Source: CAD feature listing. Evaluate the final solid. Frame: model axes, mm. Coordinates: 2 decimals unless noted, no trailing zeros. Order: outer loops, then holes, each group sorted by start corner. A loop starts at its lowest first (then second) coordinate and runs counter-clockwise, first axis right, second up.
```python
from build123d import *

# Parameters (mm, degrees)
SKETCH1_R           = 25
BOSS_EXTRUDE1_DEPTH = 3
CUT_EXTRUDE1_DEPTH  = 0.1


with BuildPart() as part:
    # Sketch1 → Boss-Extrude1 (new body)
    with BuildSketch(Plane(origin=(0, 0, 0), x_dir=(0, 1, 0), z_dir=(0, 0, 1))):
        with Locations(Location((0, 0, 0), (0, 0, 270))):
            Circle(SKETCH1_R)
    extrude(amount=BOSS_EXTRUDE1_DEPTH)

    # Sketch3 → Cut-Extrude1 (cut)
    # profile 1 of 2: a face of its own
    with BuildSketch(Plane.XY.offset(3)):
        with BuildLine():
            Line((-2.135536589, -3.91952773), (-2.135536589, -5.589026656))
            Line((-2.135536589, -5.589026656), (-9.359581237, -5.589026656))
            Line((-9.359581237, -5.589026656), (-9.359581237, -3.91952773))
            Line((-9.359581237, -3.91952773), (-6.712942094, -3.91952773))
            Line((-6.712942094, -3.91952773), (-6.712942094, 3.6938054))
            add(Edge.make_bspline(
                [(-6.712942094, 3.6938054), (-6.711155885, 3.847105408), (-6.707541754, 4.157285237), (-6.693777105, 4.467181218), (-6.686815351, 4.623917478)],
                knots=[0, 0, 0, 0, 0.98845891, 2, 2, 2, 2], degree=3))
            Line((-6.686815351, 4.623917478), (-8.565328227, 3.051087504))
            add(Edge.make_bspline(
                [(-8.565328227, 3.051087504), (-8.617759942, 3.014331802), (-8.716372329, 2.945202508), (-8.880339811, 2.88896631), (-9.036125684, 2.875345654), (-9.18237461, 2.882130045), (-9.313965386, 2.925554364), (-9.431240682, 2.977107644), (-9.527057416, 3.04704147), (-9.573128253, 3.104942057), (-9.594721931, 3.132080409)],
                knots=[0, 0, 0, 0, 1.335478134, 2.511737127, 3.574879376, 4.598514131, 5.550291057, 6.455707661, 7.276180923, 8, 8, 8, 8], degree=3))
            Line((-9.594721931, 3.132080409), (-10.297531338, 4.098769928))
            Line((-10.297531338, 4.098769928), (-6.315815589, 7.484795919))
            Line((-6.315815589, 7.484795919), (-4.484330852, 7.484795919))
            Line((-4.484330852, 7.484795919), (-4.484330852, -3.91952773))
            Line((-4.484330852, -3.91952773), (-2.135536589, -3.91952773))
        make_face()
    # profile 2 of 2: a face of its own
    with BuildSketch(Plane.XY.offset(3)):
        with BuildLine():
            add(Edge.make_bspline(
                [(9.075449156, 0.940046608), (9.071019121, 0.664701426), (9.062453061, 0.132285105), (8.994417033, -0.639500558), (8.881176325, -1.355733726), (8.722500681, -2.017311728), (8.521457839, -2.6215582), (8.285804124, -3.171554325), (8.017952132, -3.668932341), (7.711163277, -4.110013082), (7.372230822, -4.49674732), (7.00440566, -4.832496752), (6.604657821, -5.113627074), (6.176960126, -5.341859495), (5.726135225, -5.515862981), (5.257991212, -5.64302657), (4.771230439, -5.71676622), (4.440808731, -5.727356618), (4.273353654, -5.732723747)],
                knots=[0, 0, 0, 0, 1.427761042, 2.760764776, 4.014112494, 5.185114878, 6.284837347, 7.312563931, 8.284692091, 9.209319466, 10.092619187, 10.946314317, 11.785842449, 12.620313761, 13.453990262, 14.286626251, 15.131675901, 16, 16, 16, 16], degree=3))
            add(Edge.make_bspline(
                [(4.273353654, -5.732723747), (4.105903463, -5.727337226), (3.775491393, -5.716708563), (3.28949381, -5.643374433), (2.823176442, -5.515750192), (2.375519546, -5.342384412), (1.952183128, -5.113690706), (1.557547903, -4.830750182), (1.190020452, -4.497705935), (0.853943156, -4.109729476), (0.54959844, -3.66884397), (0.284444452, -3.171414662), (0.051406307, -2.621436329), (-0.146966158, -2.017182795), (-0.303219138, -1.355635346), (-0.412983668, -0.639255268), (-0.481995779, 0.132254791), (-0.490420263, 0.664691092), (-0.494777081, 0.940046608)],
                knots=[0, 0, 0, 0, 0.870312425, 1.717297107, 2.547469919, 3.378839009, 4.207245088, 5.041308741, 5.896958699, 6.779301806, 7.703466893, 8.675663034, 9.703960984, 10.804778541, 11.977405589, 13.232913505, 14.568969609, 16, 16, 16, 16], degree=3))
            add(Edge.make_bspline(
                [(-0.494777081, 0.940046608), (-0.490395372, 1.216269227), (-0.48192189, 1.750436948), (-0.413378742, 2.522881329), (-0.303182258, 3.238353368), (-0.14706114, 3.897338419), (0.051897585, 4.499634222), (0.284526412, 5.048825866), (0.54881735, 5.545984912), (0.854669604, 5.98502091), (1.190812097, 6.372527453), (1.556644922, 6.708377286), (1.952311151, 6.990983264), (2.375424524, 7.220136663), (2.823644607, 7.392411155), (3.289018042, 7.524330183), (3.775555765, 7.59656853), (4.105925113, 7.607351991), (4.273353654, 7.612816963)],
                knots=[0, 0, 0, 0, 1.435879915, 2.776748353, 4.028067345, 5.196555383, 6.293321804, 7.321852275, 8.294268251, 9.214920023, 10.097462647, 10.956354759, 11.790607013, 12.619200412, 13.450757493, 14.282314574, 15.129490778, 16, 16, 16, 16], degree=3))
            add(Edge.make_bspline(
                [(4.273353654, 7.612816963), (4.440787348, 7.607371921), (4.771166865, 7.596627784), (5.258463213, 7.523978149), (5.725669157, 7.392522252), (6.177055392, 7.219613418), (6.60452845, 6.990917769), (7.005314836, 6.710131059), (7.371436101, 6.371566293), (7.710433994, 5.985297187), (8.018735703, 5.546079999), (8.285722605, 5.048964987), (8.520961624, 4.499752358), (8.722595975, 3.897468449), (8.881140026, 3.238452128), (8.994817843, 2.52312835), (9.06237705, 1.750406214), (9.070993512, 1.216258751), (9.075449156, 0.940046608)],
                knots=[0, 0, 0, 0, 0.868519118, 1.713758561, 2.547769124, 3.381632863, 4.216291591, 5.056008275, 5.912936842, 6.796434946, 7.717566584, 8.689913077, 9.717870481, 10.813555276, 11.980430531, 13.229599676, 14.567402704, 16, 16, 16, 16], degree=3))
        make_face()
        with BuildLine():
            add(Edge.make_bspline(
                [(6.773683032, 0.940046608), (6.77138159, 1.165667325), (6.766970374, 1.598118622), (6.728307454, 2.215549989), (6.664537347, 2.773177449), (6.573734771, 3.271486255), (6.459730373, 3.715657268), (6.335426284, 4.112484148), (6.184804403, 4.459488084), (6.021296706, 4.762466776), (5.841121054, 5.020853425), (5.645543659, 5.235343664), (5.438884475, 5.411292967), (5.216254332, 5.542223154), (4.986608258, 5.638348235), (4.753221726, 5.71009288), (4.514460938, 5.753355227), (4.353647187, 5.758074514), (4.273353654, 5.760430831)],
                knots=[0, 0, 0, 0, 1.791502552, 3.433805244, 4.910094652, 6.246187574, 7.452181068, 8.550059512, 9.544407747, 10.451236363, 11.280112373, 12.038857448, 12.750772576, 13.426816362, 14.080634448, 14.723832631, 15.362815766, 16, 16, 16, 16], degree=3))
            add(Edge.make_bspline(
                [(4.273353654, 5.760430831), (4.193929125, 5.758074214), (4.034841366, 5.753353899), (3.79867417, 5.710082057), (3.567895178, 5.638325997), (3.34083945, 5.542172118), (3.120806553, 5.411186913), (2.916795755, 5.235215966), (2.723856864, 5.020694951), (2.546375935, 4.762292593), (2.385287867, 4.459402243), (2.238157676, 4.111833538), (2.112289385, 3.71612128), (2.002158784, 3.271274037), (1.913387308, 2.773117016), (1.853202684, 2.215358755), (1.813457884, 1.598145015), (1.809206893, 1.165676374), (1.806989044, 0.940046608)],
                knots=[0, 0, 0, 0, 0.632503036, 1.266906969, 1.905736897, 2.555481396, 3.22795667, 3.937072042, 4.693831014, 5.521656093, 6.428370863, 7.423497167, 8.525249946, 9.733806716, 11.073374713, 12.554077104, 14.202175365, 16, 16, 16, 16], degree=3))
            add(Edge.make_bspline(
                [(1.806989044, 0.940046608), (1.809150434, 0.713542452), (1.813277296, 0.281065434), (1.853525525, -0.336977132), (1.913149895, -0.894791395), (2.002172463, -1.393796121), (2.112305148, -1.838626066), (2.238092594, -2.234402012), (2.385500536, -2.581763606), (2.545349233, -2.884693439), (2.725631944, -3.140918115), (2.915791122, -3.357748528), (3.120931921, -3.533598875), (3.340807832, -3.664718687), (3.56790337, -3.760838431), (3.798672018, -3.832603361), (4.034841901, -3.875872898), (4.193929303, -3.88059352), (4.273353654, -3.882950289)],
                knots=[0, 0, 0, 0, 1.804043418, 3.444560704, 4.931565859, 6.27059941, 7.478674004, 8.579987218, 9.574716498, 10.481069517, 11.302874194, 12.064498727, 12.773331185, 13.445538162, 14.095023433, 14.733598488, 15.367749313, 16, 16, 16, 16], degree=3))
            add(Edge.make_bspline(
                [(4.273353654, -3.882950289), (4.353647007, -3.880593815), (4.514460398, -3.875874216), (4.753223901, -3.832614228), (4.986599988, -3.760860505), (5.21628622, -3.664770329), (5.438758244, -3.533702706), (5.646550427, -3.357890125), (5.839340697, -3.14105262), (6.022326866, -2.884880989), (6.184591644, -2.581847144), (6.335491123, -2.235053157), (6.459714851, -1.838161923), (6.573720226, -1.394008202), (6.664781663, -0.894853631), (6.727975633, -0.337166314), (6.767152111, 0.281091524), (6.771438232, 0.713551419), (6.773683032, 0.940046608)],
                knots=[0, 0, 0, 0, 0.636931218, 1.275660623, 1.918603401, 2.572161866, 3.247937206, 3.959569644, 4.723131429, 5.546035468, 6.452503996, 7.44645739, 8.543899885, 9.749414497, 11.084976877, 12.567545687, 14.202297145, 16, 16, 16, 16], degree=3))
        make_face(mode=Mode.SUBTRACT)
    extrude(amount=-CUT_EXTRUDE1_DEPTH, mode=Mode.SUBTRACT)


solid = part.part
```
1. Section query B-B, the plane x = -20. Output: boundary loops of the cut face in (y, z).
2. Section query A-A, the plane z = 1.45. Output: boundary loops of the cut face in (x, y), plus the area to 3 significant figures.
3. Contact query for a flat-ended pin moving along its axis: P1, Ø1.5, axis at x = -3, z = 1, coming from the -Y side. Output: stop coordinate, or through.
4. Section query C-C, the plane y = -9. Output: boundary loops of the cut face in (x, z).
5. Material intervals for line 1 along Y through (x, z) = (-0.5, 1.5) (3 decimals); line 2 along Z through (x, y) = (-8, 5); line 3 along X through (y, z) = (17, 2.95), sorted ascending.
6. Draft query along Y for faces 1 (the cylindrical face through (23.846, 7.509, 1.479)), 2 (the flat face through (8, 1, 2.9)), 3 (the flat face through (0, -5, 3)), 4 (the flat face through (-6, 0, 2.9)). Return one class per face: +Y half, -Y half, draft (parallel to the pull), parting line (faces both ways), or undercut.
Answer key:
1. outline: (-15, 0) - (15, 0) - (15, 3) - (-15, 3) - close
2. outline: circle Ø50 at (0, 0)
2. area: 1,960 mm2
3. P1: stops at y = -24.9
4. outline: (-23.32, 0) - (23.32, 0) - (23.32, 3) - (-23.32, 3) - close
5. line 1: y = -24.995 to 24.995
5. line 2: z = 0 to 2.9
5. line 3: x = -18.33 to 18.33
6. face 1: parting line
6. face 2: undercut
6. face 3: draft
6. face 4: undercut
